Study the drawing (mm; zero at the part's minimum x, y, z) and answer. A direction names the side the tool comes from. Round coordinates to 2 decimals unless told otherwise and drop trailing zeros. Write each loop counter-clockwise with the first axis right and the second up, starting at its lowest first coordinate (ties: lowest second). Pieces come first, ordered by that corner, then holes.
(1) For the marked faces 1 and 2, determine the directions among +Z, -Z, +X, -X, +Y, -Y from which every point of the face is accessible in a straight line to the end or side of a thin tool.
(2) A cutting plane is placed at B-B, the plane z = 5.5. Give the vertices of the cut face in (x, y) (3 decimals).
(3) Each of these flat-tipped pins is pushed along its axis until it touches: pin 1 Ø5 at (x, z) = (2.5, 12) entering from -Y; pin 2 Ø1 at (x, z) = (20.5, 9) entering from +Y; pin 3 Ø2 at (x, z) = (15.5, 12.5) entering from -Y. Where does it stop, or does it pass through?
(4) A cutting plane is placed at A-A, the plane x = 31.75. Give the vertices of the cut face in (y, z) (3 decimals), and give its area (3 significant figures).
(5) A cutting plane is placed at C-C, the plane x = 44.5. Give the vertices of the cut face in (y, z).
(6) A cutting plane is placed at D-D, the plane x = 15.5. Give the vertices of the cut face in (y, z), and give its area (3 significant figures).
(7) Find the intervals of material crossed by probe 1 along Y at (x, z) = (31.75, 13) (3 decimals); probe 2 along X at (y, z) = (25.5, 2); probe 3 along X at (y, z) = (10, 15.25), in increasing order.
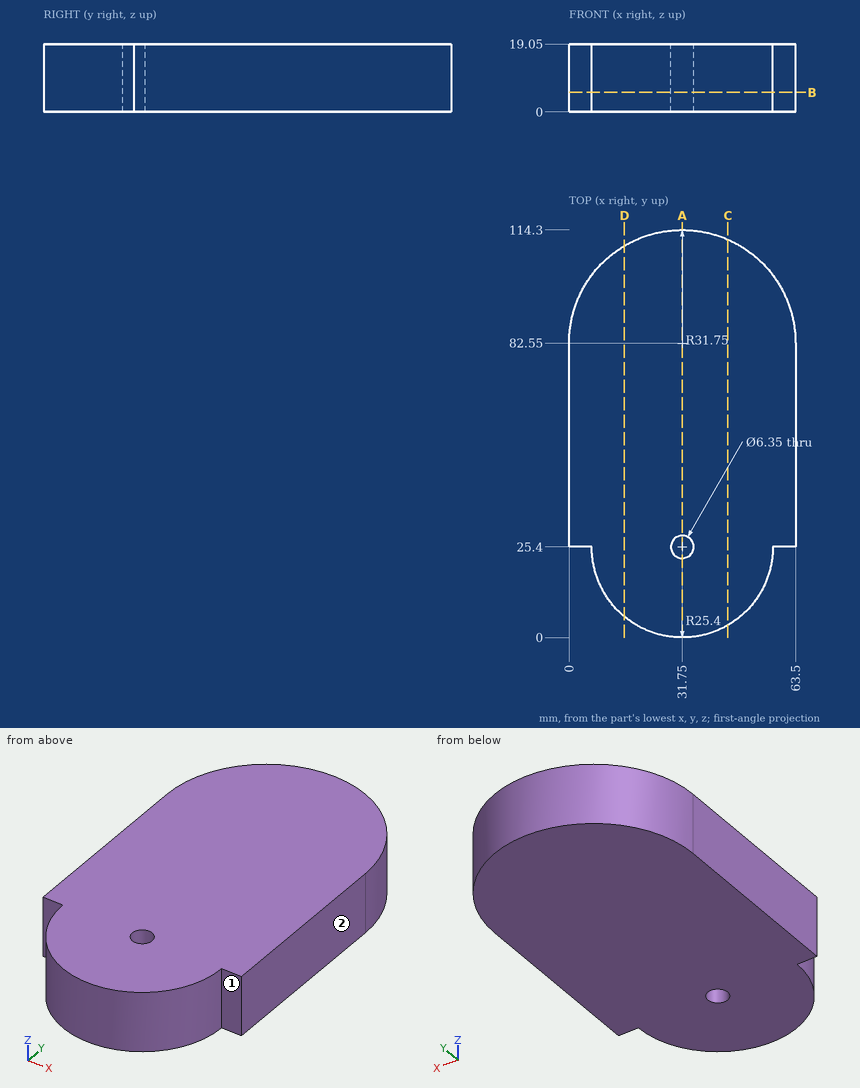
Solutions:
1. face 1: +Z, -Z, +X, -Y
1. face 2: +Z, -Z, +X, +Y, -Y
2. outline: (0, 25.4) - (6.35, 25.4) arc R25.4 ccw to (57.15, 25.4) - (63.5, 25.4) - (63.5, 82.55) arc R31.75 ccw to (0, 82.55) - close; hole circle Ø6.35 at (31.75, 25.4)
3. pin 1: stops at y = 25.4
3. pin 2: stops at y = 112.42
3. pin 3: stops at y = 5.09
4. outline: (0, 0) - (22.225, 0) - (22.225, 19.05) - (0, 19.05) - close; (28.575, 0) - (114.3, 0) - (114.3, 19.05) - (28.575, 19.05) - close
4. area: 2,060 mm2
5. outline: (3.43, 0) - (111.63, 0) - (111.63, 19.05) - (3.43, 19.05) - close
6. outline: (5.88, 0) - (109.83, 0) - (109.83, 19.05) - (5.88, 19.05) - close
6. area: 1,980 mm2
7. probe 1: y = 0 to 22.225, 28.575 to 114.3
7. probe 2: x = 0 to 28.58, 34.92 to 63.5
7. probe 3: x = 11.55 to 51.95
